from build123d import *

# Parameters (mm, degrees)
SKETCH_1_W      = 60
SKETCH_1_H      = 60
SKETCH_1_R      = 2.5
SKETCH_1_R_2    = 1.65
EXTRUDE_1_DEPTH = 4
FILLET_1_R      = 2
CHAMFER_1_SIZE  = 1.9


with BuildPart() as part:
    # Эскиз1 → Бобышка-Вытянуть1 (new body)
    with BuildSketch(Plane(origin=(0, 0, 0), x_dir=(1, 0, 0), z_dir=(0, 1, 0))):
        with Locations((-8.705299467, 3.781032797)):
            Rectangle(SKETCH_1_W, SKETCH_1_H)
        with Locations(Location((-33.454036809, 28.529770139, 0), (0, 0, 270))):
            Circle(SKETCH_1_R, mode=Mode.SUBTRACT)
        with Locations(Location((16.043437874, 28.529770139, 0), (0, 0, 270))):
            Circle(SKETCH_1_R, mode=Mode.SUBTRACT)
        with Locations(Location((-33.454036809, -20.967704544, 0), (0, 0, 270))):
            Circle(SKETCH_1_R, mode=Mode.SUBTRACT)
        with Locations(Location((16.043437874, -20.967704544, 0), (0, 0, 270))):
            Circle(SKETCH_1_R, mode=Mode.SUBTRACT)
        with Locations(Location((-33.705299467, 3.781032797, 0), (0, 0, 270))):
            Circle(SKETCH_1_R_2, mode=Mode.SUBTRACT)
        with Locations(Location((16.294700533, 3.781032797, 0), (0, 0, 270))):
            Circle(SKETCH_1_R_2, mode=Mode.SUBTRACT)
        with Locations(Location((-8.705299467, 28.781032797, 0), (0, 0, 270))):
            Circle(SKETCH_1_R_2, mode=Mode.SUBTRACT)
        with Locations(Location((-8.705299467, -21.218967203, 0), (0, 0, 270))):
            Circle(SKETCH_1_R_2, mode=Mode.SUBTRACT)
        with BuildLine():
            ThreePointArc((-27.195682571, 9.974233316), (-28.205299467, 3.781032797), (-27.195682571, -2.412167721))
            ThreePointArc((-27.195682571, -2.412167721), (-29.05264456, -16.566312295), (-14.898499986, -14.709350307))
            ThreePointArc((-14.898499986, -14.709350307), (-8.739771419, -15.718936733), (-2.577511871, -14.731131289))
            ThreePointArc((-2.577511871, -14.731131289), (11.447243796, -16.371510466), (9.806864619, -2.346754799))
            ThreePointArc((9.806864619, -2.346754799), (10.794700533, 3.781032797), (9.806864619, 9.908820393))
            ThreePointArc((9.806864619, 9.908820393), (11.447243796, 23.933576061), (-2.577511871, 22.293196884))
            ThreePointArc((-2.577511871, 22.293196884), (-8.739771419, 23.281002328), (-14.898499986, 22.271415901))
            ThreePointArc((-14.898499986, 22.271415901), (-29.05264456, 24.12837789), (-27.195682571, 9.974233316))
        make_face(mode=Mode.SUBTRACT)
    extrude(amount=EXTRUDE_1_DEPTH)

    # Скругление1
    fillet_1_edges = [part.edges().sort_by_distance(p)[0] for p in [
        (-38.705299467, 2, -33.781032797),
        (21.294700533, 2, -33.781032797),
        (21.294700533, 2, 26.218967203),
        (-38.705299467, 2, 26.218967203),
    ]]
    fillet(fillet_1_edges, radius=FILLET_1_R)

    # Фаска1
    chamfer_1_edges = [part.edges().sort_by_distance(p)[0] for p in [
        (-33.454036809, 4, -31.029770139),
        (16.043437874, 4, -31.029770139),
        (-33.454036809, 4, 18.467704544),
        (16.043437874, 4, 18.467704544),
    ]]
    chamfer(chamfer_1_edges, length=CHAMFER_1_SIZE)


solid = part.part
The model under review builds one solid part; all positions refer to its coordinate system, in mm. A direction names the side the tool comes from. Coordinates: 2 decimals unless noted, no trailing zeros. Order: outer loops, then holes, each group sorted by start corner. A loop starts at its lowest first (then second) coordinate and runs counter-clockwise, first axis right, second up. Notation, with made-up numbers: (-26.5, 51.5) -> (-5.5, 51.5) arc R12 cw to (-5.5, 70.5) -> close; hole circle Ø4 at (78, -10.75). An arc over 180 degrees is marked (long way). Answer in a Markdown table with one row per item.
(1) Consider section A-A (z = -21.5). Write out the cut boundary in (x, y).
Answers:
| item | result |
|---|---|
| outline | (-38.71, 0) -> (-30.88, 0) -> (-30.88, 4) -> (-38.71, 4) -> close; (13.18, 0) -> (21.29, 0) -> (21.29, 4) -> (13.18, 4) -> close |
(2) Consider section C-C (y = 3). State how many separate pieces and enclosed holes the cut face has, plus the area to 3 significant figures.
Answers:
| item | result |
|---|---|
| separate pieces | 1 |
| enclosed holes | 9 |
| area | 1,650 mm² |
(3) Wall thickness on line 1 along Z through (x, y) = (-28.5, 3.1); line 2 along X through (y, z) = (1.6, 16); line 3 along Z through (x, y) = (-29, 3.45): over which ranges is each line inside the solid? List them lowest first.
Answers:
| item | result |
|---|---|
| line 1 | -33.78 to -24.64, -10.89 to 3.33, 17.07 to 26.22 |
| line 2 | -38.71 to -29.57, -15.8 to -1.63, 11.8 to 21.29 |
| line 3 | -33.78 to -24.18, -11.35 to 3.79, 16.62 to 26.22 |
(4) Machinability: for faces 1 (the flat face through (-9, 2, 26.219)), 2 (the cylindrical face through (-8.83, 1.97, 15.72)), which of the approach directions +Z, -Z, +X, -X, +Y, -Y give a long, thin tool a straight path to every point of the face, cutting with its end or side? Answer none if there is none.
Answers:
| item | result |
|---|---|
| face 1 | +Z, +X, -X, +Y, -Y |
| face 2 | +Y, -Y |
(5) Insertion check: pin 1 (6.5 mm diameter, centred on x = 16.04, z = -28.53, fed in from +Y); pin 2 (8 mm diameter, centred on x = -33.45, z = -28.53, fed in from +Y). Each pin has a flat end and moves straight along its axis. Give the tip position at first contact, or say it passes through.
Answers:
| item | result |
|---|---|
| pin 1 | y = 2.85 |
| pin 2 | y = 3.6 |
(6) The part is to be moulded in two halves that separate along Z. For faces 3 (the flat face through (21.295, 2, -3)), 4 (the cylindrical face through (-35.895, 1.035, -29.072)), 5 (the flat face through (-9, 2, -33.781)), 6 (the cylindrical face through (-35.672, 1.035, 22.121)), say which applies: +Z half, -Z half, draft (parallel to the pull), parting line (faces both ways), or undercut.
Answers:
| item | result |
|---|---|
| face 3 | draft |
| face 4 | undercut |
| face 5 | -Z half |
| face 6 | undercut |
(7) Consider section B-B (x = -24). Write out the cut boundary in (y, z), plus the area to 3 significant figures.
Answers:
| item | result |
|---|---|
| outline | (0, -33.78) -> (4, -33.78) -> (4, -26.67) -> (0, -26.67) -> close; (0, 19.11) -> (4, 19.11) -> (4, 26.22) -> (0, 26.22) -> close |
| area | 56.9 mm² |
